Here's how the part is built. I have some questions about the finished solid (model axes, mm). A direction names the side the tool comes from. Coordinates: 2 decimals unless noted, no trailing zeros. Write each loop counter-clockwise with the first axis right and the second up, starting at its lowest first coordinate (ties: lowest second). Pieces come first, ordered by that corner, then holes. Notation, with made-up numbers: M 22,50.25 L 69,50.25 A15 cw 69,59.25 Z; hole C 12.5,33.5 d1. An arc over 180 degrees is marked long. Use one line per item in the form item = value. Start each with the question number.
1. I want a section at B-B, the plane x = 720. List the corners of the cut face in (y, z) for me.
2. On a 3-axis mill with a long thin cutter (end or side, diameter ignored), from which of +Z, -Z, +X, -X, +Y, -Y can I reach the whole of each face in a straight line? I mean faces 1 (the face through (-1000, -13, 51)), 2 (the face through (-87, -958, 0)). Say none if no direction works.
3. I want a section at A-A, the plane y = -783.5. List the corners of the cut face in (x, z) for me, plus the area to 3 significant figures.
4. I want a section at C-C, the plane z = 17.5. List the corners of the cut face in (x, y) for me.
5. Please list where these lines run through material, in increasing order: line 1 along X through (y, z) = (271, 87); line 2 along Y through (x, z) = (-937, 43.5). Write a range as [from, to].
from build123d import *

# Parameters (mm, degrees)
F0_W     = 2400
F0_H     = 2200
F1_DEPTH = 100
F2_W     = 2400
F2_H     = 2200
F2_W_2   = 2200
F2_H_2   = 2000
F3_DEPTH = 100.001
F2_W_3   = 2000
F2_H_3   = 1800
F4_DEPTH = 100.001


with BuildPart() as f1:
    # F0 (on Top) → F1 (new body)
    with BuildSketch(Plane.XY):
        Rectangle(F0_W, F0_H)
    extrude(amount=F1_DEPTH)

    # F2 (on face) → F3 (cut, through all)
    with BuildSketch(Plane.XY.offset(100)):
        Rectangle(F2_W, F2_H)
        Rectangle(F2_W_2, F2_H_2, mode=Mode.SUBTRACT)
    extrude(amount=-F3_DEPTH, mode=Mode.SUBTRACT)

    # F2 (on face) → F4 (cut, through all)
    with BuildSketch(Plane.XY.offset(100)):
        Rectangle(F2_W_3, F2_H_3)
    extrude(amount=-F4_DEPTH, mode=Mode.SUBTRACT)


solid = f1.part
Answer list:
q1.outline = M -1000,0 L -900,0 L -900,100 L -1000,100 Z; M 900,0 L 1000,0 L 1000,100 L 900,100 Z
q2.face_1 = +Z, -Z
q2.face_2 = -Z, +X, -X, +Y, -Y
q3.outline = M -1100,0 L -1000,0 L -1000,100 L -1100,100 Z; M 1000,0 L 1100,0 L 1100,100 L 1000,100 Z
q3.area = 20,000 mm²
q4.outline = M -1100,-1000 L 1100,-1000 L 1100,1000 L -1100,1000 Z; hole M -1000,-900 L 1000,-900 L 1000,900 L -1000,900 Z
q5.line_1 = [-1100, -1000], [1000, 1100]
q5.line_2 = [-1000, -900], [900, 1000]
